Input: part model. Units: mm. Frame: model coordinates. Give positions to 0.01 mm unless a question says otherwise; leave off trailing zeros. Order: outer loops, then holes, each group sorted by start corner. A loop starts at its lowest first (then second) coordinate and runs counter-clockwise, first axis right, second up. Notation, with made-up numbers: (76.25, 54.5) - (102.25, 54.5) arc R16 ccw to (102.25, 62.5) - close; hole circle Ø1 at (39, 16). An arc over 180 degrees is marked (long way). Answer in a Markdown table with one row per item. Add a question column.
1. Ray query, line 1 (Y direction, x = 36.83, z = 13); line 2 (Y direction, x = -36.83, z = 23); line 3 (X direction, y = -29, z = 11). Return the intervals inside material, ascending. Write a range as [from, to].
2. Section query A-A on x = -36.83. Return loops of the section in (y, z), and give its area (3 significant figures).
3. Contact query for a flat-ended pin moving along its axis: pin 1 (1.3 mm diameter, centred on x = -36.5, y = -35, fed in from +Z). Output: stop coordinate, or through.
4. Section query B-B on y = -27.94. Return loops of the section in (x, z).
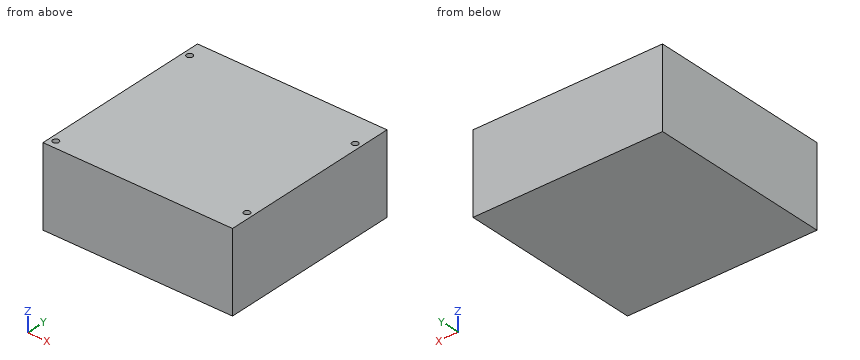
```python
from build123d import *

# Parameters (mm, degrees)
SKETCH1_W           = 78.74
SKETCH1_H           = 76.2
SKETCH1_R           = 1.27
BOSS_EXTRUDE1_DEPTH = 33.02
SKETCH2_R           = 1.27
BOSS_EXTRUDE2_DEPTH = 2.54
SKETCH3_R           = 1.27
BOSS_EXTRUDE3_DEPTH = 2.54


with BuildPart() as part:
    # Sketch1 → Boss-Extrude1 (new body)
    with BuildSketch(Plane.XY):
        Rectangle(SKETCH1_W, SKETCH1_H)
        with Locations((36.83, 25.4)):
            Circle(SKETCH1_R, mode=Mode.SUBTRACT)
        with Locations((36.83, -27.94)):
            Circle(SKETCH1_R, mode=Mode.SUBTRACT)
        with Locations((-36.83, 31.242)):
            Circle(SKETCH1_R, mode=Mode.SUBTRACT)
        with Locations((-36.83, -34.798)):
            Circle(SKETCH1_R, mode=Mode.SUBTRACT)
    extrude(amount=BOSS_EXTRUDE1_DEPTH)

    # Sketch2 → Boss-Extrude2 (add)
    with BuildSketch(Plane(origin=(0, 0, 0), x_dir=(-1, 0, 0), z_dir=(0, 0, -1))):
        with Locations((-36.83, 25.4)):
            Circle(SKETCH2_R)
    extrude(amount=-BOSS_EXTRUDE2_DEPTH)

    # Sketch3 → Boss-Extrude3 (add)
    with BuildSketch(Plane(origin=(0, 0, 0), x_dir=(-1, 0, 0), z_dir=(0, 0, -1))):
        with Locations((36.83, 31.242)):
            Circle(SKETCH3_R)
        with Locations((36.83, -34.798)):
            Circle(SKETCH3_R)
        with Locations((-36.83, -27.94)):
            Circle(SKETCH3_R)
    extrude(amount=-BOSS_EXTRUDE3_DEPTH)


solid = part.part
```
Answer:
| question | item | result |
|---|---|---|
| 1 | line 1 | y = [-38.1, -29.21], [-26.67, 24.13], [26.67, 38.1] |
| 1 | line 2 | y = [-38.1, -36.07], [-33.53, 29.97], [32.51, 38.1] |
| 1 | line 3 | x = [-39.37, 36.13], [37.53, 39.37] |
| 2 | outline | (-38.1, 0) - (38.1, 0) - (38.1, 33.02) - (32.51, 33.02) - (32.51, 2.54) - (29.97, 2.54) - (29.97, 33.02) - (-33.53, 33.02) - (-33.53, 2.54) - (-36.07, 2.54) - (-36.07, 33.02) - (-38.1, 33.02) - close |
| 2 | area | 2,360 mm² |
| 3 | pin 1 | stops at z = 2.54 |
| 4 | outline | (-39.37, 0) - (39.37, 0) - (39.37, 33.02) - (38.1, 33.02) - (38.1, 2.54) - (35.56, 2.54) - (35.56, 33.02) - (-39.37, 33.02) - close |
